Autodesk Fusion 360 part; units mm, degrees
sketch "Sketch1" plane through (0, 0, 0) normal (0, 1, 0) x (1, 0, 0)
  circle A0 centre (0, -6.35) radius 5.0165
  dimension "d1" = 10.033
extrude "Extrude1" add sketch "Sketch1" along normal blind 57.785
hole "Hole1" at (0, 55.245, 11.3665) direction (0, 0, -1) diameter 2.54 depth 19.05 tip angle 118
extrude "Extrude2" cut 1 faces at (-0.3721, 0, 4.7198) along direction (0, 1, 0) blind 2.54
sketch "Sketch3" plane through (0, 2.54, 0) normal (0, -1, 0) x (1, 0, 0)
  circle A0 centre (0, 6.35) radius 5.0165
  line L0 (-2.54, 8.89) -> (2.54, 8.89)
  line L1 (2.54, 8.89) -> (2.54, 3.81)
  line L2 (2.54, 3.81) -> (-2.54, 3.81)
  line L3 (-2.54, 3.81) -> (-2.54, 8.89)
extrude "Extrude3" add sketch "Sketch3" along normal blind 2.54 contours L0 L1 L2 L3
extrude "Extrude4" add 1 faces at (0.8467, 0.8467, 8.89) along direction (0, 0, 1) blind 3.302
extrude "Extrude5" add 1 faces at (2.54, 0.8467, 8.8926) along direction (1, 0, 0) blind 3.302
extrude "Extrude6" add 1 faces at (2.5426, 0.8467, 3.81) along direction (0, 0, -1) blind 3.302
extrude "Extrude7" add 1 faces at (-2.54, 0.8467, 4.908) along direction (-1, 0, 0) blind 3.302
fillet "Fillet1" radius 5.842 4 edges at (-5.842, 1.27, 12.192) (5.842, 1.27, 12.192) (5.842, 1.27, 0.508) (-5.842, 1.27, 0.508)
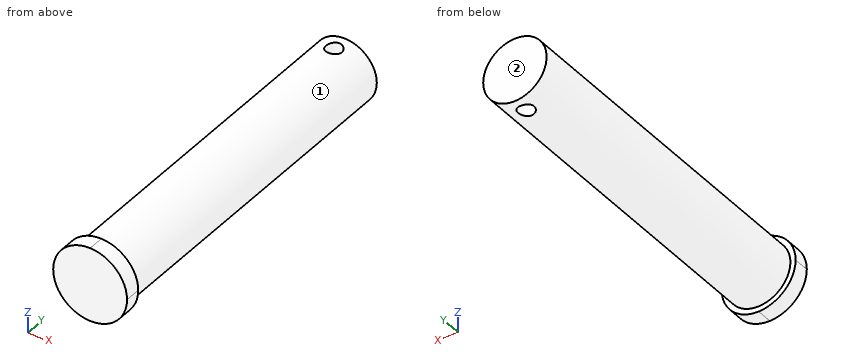
Check sheet for the modelled part. Datum: model origin and axes. Units: mm. Face numbers are marked on the shaded views. A direction names the side the tool comes from. Round coordinates to 2 decimals unless told otherwise and drop trailing zeros. Loops run counter-clockwise (first coordinate to the right, second up) from the corner with the lowest first, then second, coordinate; pieces in that order, holes last. Notation, with made-up numbers: M 85,-29.75 L 142,-29.75 A15 cw 142,-8.75 Z; hole C 0.5,81.5 d9. An arc over 180 degrees is marked long. Answer as a JSON object with one key per item and string values.
1. Section check C-C (y = 45). Record the boundary of the cut face in (x, z).
Reply:
{"outline": "C 0,6.35 d10.03"}
2. Section check D-D (z = 3). Record the boundary of the cut face in (x, y) (3 decimals).
Reply:
{"outline": "M -4.787,0 L 4.787,0 L 4.787,2.54 L 3.734,2.54 L 3.734,57.785 L -3.734,57.785 L -3.734,2.54 L -4.787,2.54 Z; hole C 0,55.245 d2.54"}
3. Section check A-A (z = 10.75). Record the boundary of the cut face in (x, y) (3 decimals), plus the area to 3 significant figures.
Reply:
{"outline": "M -3.844,0 L 3.844,0 L 3.844,2.54 L 2.409,2.54 L 2.409,57.785 L -2.409,57.785 L -2.409,2.54 L -3.844,2.54 Z; hole C 0,55.245 d2.54", "area": "281 mm²"}
4. Gauge pin test, flat ends, axial feed: P1, Ø1.5, axis at y = 27, z = 4, coming from the +X side; P2, Ø5, axis at y = 46.5, z = 10, coming from the +X side; P3, Ø2, axis at x = -2, z = 10, coming from the -Y side; P4, Ø5, axis at x = -2.5, y = 21.5, coming from the -Z side. Record the tip position at first contact, or that the pin passes through.
Reply:
{"P1": "stops at x = 4.75", "P2": "stops at x = 4.88", "P3": "stops at y = 0", "P4": "stops at z = 1.33"}
5. Scan lines: line 1 (Y direction, x = 0, z = 6) (3 decimals); line 2 (Y direction, x = 5, z = 8.25); line 3 (Y direction, x = 0.5, z = 10.5) (3 decimals). Record each from-to range of solid material in increasing order.
Reply:
{"line 1": "y = 0 to 53.975, 56.515 to 57.785", "line 2": "y = 0 to 2.54", "line 3": "y = 0 to 54.078, 56.412 to 57.785"}
6. Section check B-B (x = 3). Record the boundary of the cut face in (y, z) (3 decimals), plus the area to 3 significant figures.
Reply:
{"outline": "M 0,1.337 L 2.54,1.337 L 2.54,2.329 L 57.785,2.329 L 57.785,10.371 L 2.54,10.371 L 2.54,11.363 L 0,11.363 Z", "area": "470 mm²"}
7. Access from +Z, -Z, +X, -X, +Y, -Y to the whole of each face (thin tool, end or side, straight path). Record for the marked faces 1 and 2.
Reply:
{"face 1": "+Y", "face 2": "+Z, -Z, +X, -X, +Y"}
